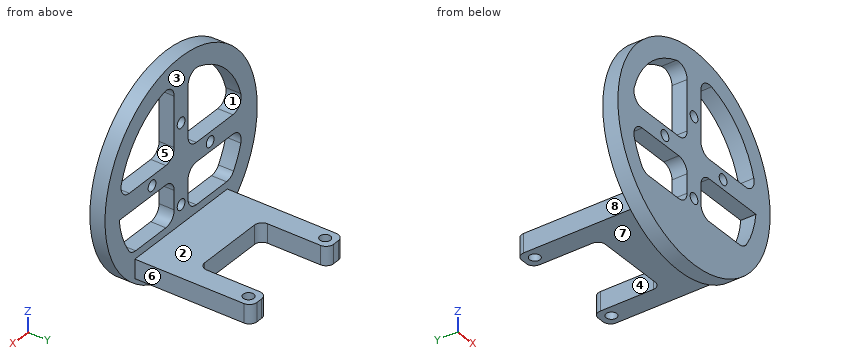
from build123d import *

# Parameters (mm, degrees)
SKETCH1_R           = 1.4
BOSS_EXTRUDE1_DEPTH = 2.5
SKETCH2_R           = 27.5
SKETCH2_R_2         = 1.4
BOSS_EXTRUDE2_DEPTH = 4
FILLET1_R           = 3
FILLET2_R           = 2


with BuildPart() as part:
    # Sketch1 → Boss-Extrude1 (new, symmetric)
    with BuildSketch(Plane.XY):
        Polygon((-16.7, 0), (16.7, 0), (16.7, 30.85), (11, 30.85), (11, 12.85), (-11, 12.85), (-11, 30.85), (-16.7, 30.85), align=None)
        with Locations((13.85, 28)):
            Circle(SKETCH1_R, mode=Mode.SUBTRACT)
        with Locations(Location((-13.85, 28, 0), (0, 0, 180))):
            Circle(SKETCH1_R, mode=Mode.SUBTRACT)
    extrude(amount=BOSS_EXTRUDE1_DEPTH, both=True)

    # Sketch2 → Boss-Extrude2 (add)
    with BuildSketch(Plane(origin=(0, 0, 0), x_dir=(1, 0, 0), z_dir=(0, 1, 0))):
        with Locations(Location((0, -18, 0), (0, 0, 270))):
            Circle(SKETCH2_R)
        with Locations(Location((0, -7.5, 0), (0, 0, 270))):
            Circle(SKETCH2_R_2, mode=Mode.SUBTRACT)
        with Locations(Location((10.5, -18, 0), (0, 0, 270))):
            Circle(SKETCH2_R_2, mode=Mode.SUBTRACT)
        with Locations(Location((0, -28.5, 0), (0, 0, 270))):
            Circle(SKETCH2_R_2, mode=Mode.SUBTRACT)
        with Locations(Location((-10.5, -18, 0), (0, 0, 270))):
            Circle(SKETCH2_R_2, mode=Mode.SUBTRACT)
        with BuildLine():
            Line((-18, -4.5), (-2.5, -4.5))
            Line((-2.5, -4.5), (-2.5, -15.5))
            Line((-2.5, -15.5), (-22.360679775, -15.5))
            ThreePointArc((-22.360679775, -15.5), (-20.916407865, -9.708203932), (-18, -4.5))
        make_face(mode=Mode.SUBTRACT)
        with BuildLine():
            Line((2.5, -4.5), (2.5, -15.5))
            Line((2.5, -15.5), (22.360679775, -15.5))
            ThreePointArc((22.360679775, -15.5), (20.916407865, -9.708203932), (18, -4.5))
            Line((18, -4.5), (2.5, -4.5))
        make_face(mode=Mode.SUBTRACT)
        with BuildLine():
            Line((-22.360679775, -20.5), (-2.5, -20.5))
            Line((-2.5, -20.5), (-2.5, -40.360679775))
            ThreePointArc((-2.5, -40.360679775), (-15.909902577, -33.909902577), (-22.360679775, -20.5))
        make_face(mode=Mode.SUBTRACT)
        with BuildLine():
            Line((2.5, -20.5), (2.5, -40.360679775))
            ThreePointArc((2.5, -40.360679775), (15.909902577, -33.909902577), (22.360679775, -20.5))
            Line((22.360679775, -20.5), (2.5, -20.5))
        make_face(mode=Mode.SUBTRACT)
    extrude(amount=-BOSS_EXTRUDE2_DEPTH)

    # Fillet1
    fillet1_edges = [part.edges().sort_by_distance(p)[0] for p in [
        (-18, -2, 4.5),
        (-22.360679775, -2, 15.5),
        (-2.5, -2, 15.5),
        (-22.360679775, -2, 20.5),
        (-2.5, -2, 40.360679775),
        (18, -2, 4.5),
        (2.5, -2, 4.5),
        (2.5, -2, 40.360679775),
        (22.360679775, -2, 20.5),
        (-2.5, -2, 4.5),
        (-2.5, -2, 20.5),
        (2.5, -2, 15.5),
        (2.5, -2, 20.5),
    ]]
    fillet(fillet1_edges, radius=FILLET1_R)

    # Fillet2
    fillet2_edges = [part.edges().sort_by_distance(p)[0] for p in [
        (-16.7, 30.85, 0),
        (-11, 30.85, 0),
        (-11, 12.85, 0),
        (11, 12.85, 0),
        (11, 30.85, 0),
        (16.7, 30.85, 0),
    ]]
    fillet(fillet2_edges, radius=FILLET2_R)


solid = part.part
Can you work these out from the model? Positions are in its coordinate system, mm. Face numbers are marked on the shaded views. A direction names the side the tool comes from. Coordinates: 2 decimals unless noted, no trailing zeros. Order: outer loops, then holes, each group sorted by start corner. A loop starts at its lowest first (then second) coordinate and runs counter-clockwise, first axis right, second up. Notation, with made-up numbers: (74.25, 44.5) -> (90.25, 44.5) arc R15 cw to (90.25, 59.5) -> close; hole circle Ø9 at (-31.5, 71). An arc over 180 degrees is marked (long way). Use one line per item in the form item = value.
Q1. Imagine slicing it at C-C, the plane x = 14. List the corners of the cut face in (y, z) for me, then the cut area to 3 significant figures.
From the geometry:
outline = (-4, -5.67) -> (0, -5.67) -> (0, -2.5) -> (26.61, -2.5) -> (26.61, 2.5) -> (0, 2.5) -> (0, 4.5) -> (-4, 4.5) -> close; (-4, 15.5) -> (0, 15.5) -> (0, 20.5) -> (-4, 20.5) -> close; (-4, 35.61) -> (0, 35.61) -> (0, 41.67) -> (-4, 41.67) -> close; (29.39, -2.5) -> (30.85, -2.5) -> (30.85, 2.5) -> (29.39, 2.5) -> close
area = 225 mm²
Q2. We'd pull the mould along Z, two halves only. Please class the marked faces 1, 2 and 3: released by +Z, released by -Z, zero draft, split by the parting line, or undercut.
From the geometry:
face_1 = undercut
face_2 = released by +Z
face_3 = zero draft
Q3. Imagine slicing it at B-B, the plane y = 28. List the corners of the cut face in (x, z) for me.
From the geometry:
outline = (-16.7, -2.5) -> (-15.25, -2.5) -> (-15.25, 2.5) -> (-16.7, 2.5) -> close; (-12.45, -2.5) -> (-11, -2.5) -> (-11, 2.5) -> (-12.45, 2.5) -> close; (11, -2.5) -> (12.45, -2.5) -> (12.45, 2.5) -> (11, 2.5) -> close; (15.25, -2.5) -> (16.7, -2.5) -> (16.7, 2.5) -> (15.25, 2.5) -> close
Q4. I need wall thicknesses on L1, parallel to X at y = -3, z = 18; L2, parallel to Z at x = 4, y = -1.5; L3, parallel to X at y = 22.5, z = -1. Which ranges of each line are inside material? Lowest first, please.
From the geometry:
L1 = -27.5 to -11.9, -9.1 to 9.1, 11.9 to 27.5
L2 = -9.21 to 4.9, 15.1 to 20.9, 39.31 to 45.21
L3 = -16.7 to -11, 11 to 16.7
Q5. Imagine slicing it at D-D, the plane z = 28.5. List the corners of the cut face in (x, y) for me, then the cut area to 3 significant figures.
From the geometry:
outline = (-25.42, -4) -> (-19.9, -4) -> (-19.9, 0) -> (-25.42, 0) -> close; (-2.5, -4) -> (-1.4, -4) -> (-1.4, 0) -> (-2.5, 0) -> close; (1.4, -4) -> (2.5, -4) -> (2.5, 0) -> (1.4, 0) -> close; (19.9, -4) -> (25.42, -4) -> (25.42, 0) -> (19.9, 0) -> close
area = 52.9 mm²
Q6. Imagine slicing it at A-A, the plane y = 16.5. List the corners of the cut face in (x, z) for me, then the cut area to 3 significant figures.
From the geometry:
outline = (-16.7, -2.5) -> (-11, -2.5) -> (-11, 2.5) -> (-16.7, 2.5) -> close; (11, -2.5) -> (16.7, -2.5) -> (16.7, 2.5) -> (11, 2.5) -> close
area = 57.0 mm²
Q7. Which directions (+Z, -Z, +X, -X, +Y, -Y) give clear straight access to the entire face, cutting with the end or side of a thin tool? Please do the marked faces 4, 5, 6, 7 and 8.
From the geometry:
face_4 = +Z, -Z, +Y
face_5 = +Y, -Y
face_6 = +Z, -Z, +X, +Y
face_7 = -Z, +X, -X, +Y
face_8 = +Z, -Z, -X, +Y
Q8. Will these pins go through, and if not, where does the flat tip stop? P1, Ø3, axis at x = 16.5, y = -1, coming from the -Z side; P2, Ø4, axis at y = 2.5, z = 22.5, coming from the -X side; P3, Ø3, axis at y = -2.5, z = 32.5, coming from the -X side; P4, Ø1.2, axis at x = 14.5, y = -2.5, coming from the +Z side.
From the geometry:
P1 = -5.05
P2 = through
P3 = -24.23
P4 = 41.73
